Autodesk Inventor part; units mm, degrees
ref_plane "作業平面1" through (-36, -24, 0) normal (0, 0, 1) x (1, 0, 0)
ref_plane "作業平面2" through (-39.3, -27.3, -10) normal (0, 0, 1) x (1, 0, 0)
ref_plane "作業平面3" through (-36, -24, -2) normal (0, 0, -1) x (0, 1, 0)
sketch "スケッチ1" plane through (0, 0, 0) normal (0, 0, 1) x (1, 0, 0)
  line L0 (36, 24) -> (36, -24) construction
  line L1 (-36, 24) -> (36, 24) construction
  line L2 (-36, -24) -> (-36, 24) construction
  line L3 (36, -24) -> (-36, -24) construction
  circle A0 centre (-33, 21) radius 1.5 construction
  circle A1 centre (-33, -21) radius 1.5 construction
  circle A2 centre (33, 21) radius 1.5 construction
  circle A3 centre (33, -21) radius 1.5 construction
  line L4 (-36.3, 24.3) -> (36.3, 24.3)
  line L5 (36.3, 24.3) -> (36.3, -24.3)
  line L6 (36.3, -24.3) -> (-36.3, -24.3)
  line L7 (-36.3, -24.3) -> (-36.3, 24.3)
  circle A4 centre (-33, -21) radius 1.6
  circle A5 centre (-33, 21) radius 1.6
  circle A6 centre (33, -21) radius 1.6
  circle A7 centre (33, 21) radius 1.6
  line L8 (-39.3, 27.3) -> (39.3, 27.3)
  line L9 (39.3, 27.3) -> (39.3, -27.3)
  line L10 (39.3, -27.3) -> (-39.3, -27.3)
  line L11 (-39.3, -27.3) -> (-39.3, 27.3)
  line L12 (-36.3, -14.3) -> (-26.3, -14.3)
  line L13 (-26.3, -14.3) -> (-26.3, -24.3)
  line L14 (-55.02, 0) -> (55.02, 0) construction
  line L15 (0, -38.22) -> (0, 38.22) construction
  line L16 (-36.3, 14.3) -> (-26.3, 14.3)
  line L17 (-26.3, 14.3) -> (-26.3, 24.3)
  line L18 (36.3, -14.3) -> (26.3, -14.3)
  line L19 (26.3, -14.3) -> (26.3, -24.3)
  line L20 (26.3, 14.3) -> (26.3, 24.3)
  line L21 (36.3, 14.3) -> (26.3, 14.3)
  line L22 (22, 5) -> (29, 5) construction
  line L23 (29, -5) -> (22, -5) construction
  line L24 (36, 24) -> (36, -24)
  line L25 (36, -24) -> (-36, -24)
  line L26 (-36, -24) -> (-36, 24)
  line L27 (-36, 24) -> (36, 24)
  circle A8 centre (-33, 21) radius 1.5
  circle A9 centre (-33, -21) radius 1.5
  circle A10 centre (33, 21) radius 1.5
  circle A11 centre (33, -21) radius 1.5
  line L28 (39.3, 5) -> (36.3, 5)
  line L29 (39.3, -5) -> (36.3, -5)
  circle A12 centre (33, 21) radius 3
  circle A13 centre (33, -21) radius 3
  circle A14 centre (-33, 21) radius 3
  circle A15 centre (-33, -21) radius 3
  point P0 (0, 0)
  dimension "d0" = 0.3
  dimension "d1" = 3.2
  dimension "d2" = 3
  dimension "d7" = 10
  dimension "d16" = 6
extrude "押し出し1" add sketch "スケッチ1" along normal blind 7 and the other way blind 3 contours L7 L6 L5 L29 L9 L10 L11 L8 L28 L4 | L28 L9 L29 L5
ref_plane "作業平面1" through (-36, -24, 0) normal (0, 0, 1) x (1, 0, 0)
extrude "押し出し3" add sketch "スケッチ1" against normal up to surface (7 mm away) from surface at 7 contours L4 L17 L27 L26 L16 L7 | L4 L5 L21 L24 L27 L20 | L17 L16 L26 A14 L27 | L12 L26 L25 L13 L6 L7 | L27 A12 L24 L21 L20 | A14 L26 L27 | A14 | L12 L13 L25 A15 L26 | L27 L24 A12 | A12 | A15 L25 L26 | A15 | L19 L25 L24 L18 L5 L6 | L24 A13 L25 L19 L18 | A13 | L24 L25 A13
extrude "押し出し4" add sketch "スケッチ1" along normal blind 3 from surface at 7 contours L7 L6 L5 L29 L9 L10 L11 L8 L28 L4 | L4 L17 L27 L26 L16 L7 | L4 L20 L27 L17 | L16 L26 L12 L7 | L4 L5 L21 L24 L27 L20 | L27 L20 L21 L24 L18 L19 L25 L13 L12 L26 L16 L17 | L17 L16 L26 A14 L27 | L12 L26 L25 L13 L6 L7 | L27 A12 L24 L21 L20 | A14 L26 L27 | A14 | L12 L13 L25 A15 L26 | L5 L18 L24 L21 | L27 L24 A12 | A12 | L13 L25 L19 L6 | A15 L25 L26 | A15 | L28 L9 L29 L5 | L19 L25 L24 L18 L5 L6 | L24 A13 L25 L19 L18 | A13 | L24 L25 A13
ref_plane "作業平面2" through (-39.3, -27.3, -10) normal (0, 0, 1) x (1, 0, 0)
ref_plane "作業平面3" through (-36, -24, -2) normal (0, 0, -1) x (0, 1, 0)
sketch "スケッチ4" plane through (0, 0, 0) normal (0, 0, 1) x (1, 0, 0)
  line L0 (36.3, 24.3) -> (36.3, -24.3)
  line L1 (39.3, 27.3) -> (39.3, -27.3)
  line L2 (39.3, 5) -> (36.3, 5)
  line L3 (39.3, -5) -> (36.3, -5)
  point P0 (0, 0)
extrude "押し出し5" cut sketch "スケッチ4" along normal up to surface (8 mm away) from surface at -10
sketch "スケッチ5" plane through (-39.3, -27.3, 10) normal (0, 0, 1) x (1, 0, 0)
  circle A0 centre (6.3, 6.3) radius 3
  circle A1 centre (72.3, 6.3) radius 3
  circle A2 centre (72.3, 48.3) radius 3
  circle A3 centre (6.3, 48.3) radius 3
  line L0 (0, 0) -> (0, 54.6)
  line L1 (78.6, 0) -> (0, 0)
  line L2 (78.6, 54.6) -> (78.6, 0)
  line L3 (0, 54.6) -> (78.6, 54.6)
  circle A4 centre (72.3, 6.3) radius 1.6
  circle A5 centre (6.3, 6.3) radius 1.6
  circle A6 centre (6.3, 48.3) radius 1.6
  circle A7 centre (72.3, 48.3) radius 1.6
  point P0 (39.3, 27.3)
extrude "押し出し6" add sketch "スケッチ5" along normal blind 5 contours L0 L3 L2 L1
fillet "フィレット1" radius 5 4 edges at (-39.3, 27.3, 6) (-39.3, -27.3, 6) (39.3, 27.3, 6) (39.3, -27.3, 6)
properties part number "enclosure"
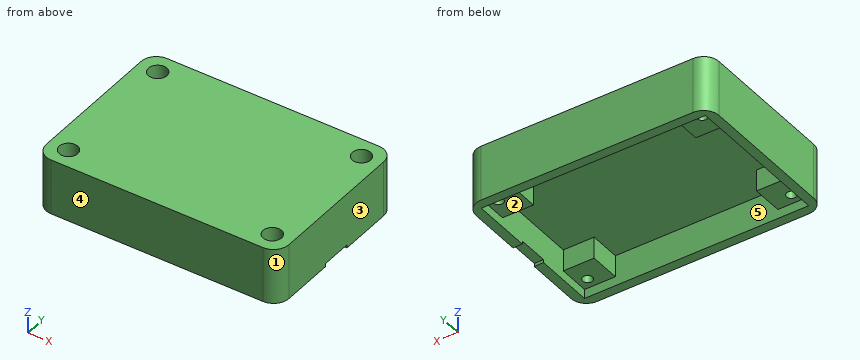
Part model, mm, in its own coordinate system. Face numbers are marked on the shaded views. A direction names the side the tool comes from. Coordinates: 2 decimals unless noted, no trailing zeros. Order: outer loops, then holes, each group sorted by start corner. A loop starts at its lowest first (then second) coordinate and runs counter-clockwise, first axis right, second up. Notation, with made-up numbers: M 88.25,1.25 L 118.25,1.25 A23 ccw 118.25,32.25 Z; hole C -10.5,43.25 d10. An arc over 180 degrees is marked long. Use a Markdown table: item, result.
(1) Cut at D-D on z = 13.75. Write the cut outline in (x, y), then the cut area to 3 significant figures.
A:
| item | result |
|---|---|
| outline | M -39.3,-22.3 A5 ccw -34.3,-27.3 L 34.3,-27.3 A5 ccw 39.3,-22.3 L 39.3,22.3 A5 ccw 34.3,27.3 L -34.3,27.3 A5 ccw -39.3,22.3 Z; hole C -33,-21 d6; hole C -33,21 d6; hole C 33,-21 d6; hole C 33,21 d6 |
| area | 4,160 mm^2 |
(2) Cut at C-C on x = 33. Write the cut outline in (y, z), then the cut area to 3 significant figures.
A:
| item | result |
|---|---|
| outline | M -27.3,-3 L -24.3,-3 L -24.3,0 L -22.6,0 L -22.6,10 L -24,10 L -24,15 L -27.3,15 Z; M -19.4,0 L -14.3,0 L -14.3,7 L 14.3,7 L 14.3,0 L 19.4,0 L 19.4,10 L 18,10 L 18,15 L -18,15 L -18,10 L -19.4,10 Z; M 22.6,0 L 24.3,0 L 24.3,-3 L 27.3,-3 L 27.3,15 L 24,15 L 24,10 L 22.6,10 Z |
| area | 513 mm^2 |
(3) Cut at B-B on z = 2.75. Write the cut outline in (x, y).
A:
| item | result |
|---|---|
| outline | M -39.3,-22.3 A5 ccw -34.3,-27.3 L 34.3,-27.3 A5 ccw 39.3,-22.3 L 39.3,22.3 A5 ccw 34.3,27.3 L -34.3,27.3 A5 ccw -39.3,22.3 Z; hole M -36.3,-14.3 L -26.3,-14.3 L -26.3,-24.3 L 26.3,-24.3 L 26.3,-14.3 L 36.3,-14.3 L 36.3,14.3 L 26.3,14.3 L 26.3,24.3 L -26.3,24.3 L -26.3,14.3 L -36.3,14.3 Z; hole C -33,-21 d3.2; hole C -33,21 d3.2; hole C 33,-21 d3.2; hole C 33,21 d3.2 |
(4) Probe L1, parallel to Y at x = -33, z = 6.25; L2, parallel to Y at x = 33, z = 13.1; L3, parallel to Y at x = -7.5, z = 5. List the from-to ranges inside material, lowest first.
A:
| item | result |
|---|---|
| L1 | y = -27.3 to -22.6, -19.4 to -14.3, 14.3 to 19.4, 22.6 to 27.3 |
| L2 | y = -27.3 to -24, -18 to 18, 24 to 27.3 |
| L3 | y = -27.3 to -24.3, 24.3 to 27.3 |
(5) Tool access for the marked faces 1 and 2: list every direction of +Z, -Z, +X, -X, +Y, -Y with a clear straight run to the whole face (end or side of a thin tool).
A:
| item | result |
|---|---|
| face 1 | +Z, -Z, +X, -Y |
| face 2 | -Z |
(6) Pull direction X, two halves, no side cores. Call the marked faces 3, 4 and 5: released by +X, released by -X, zero draft, split by the parting line, or undercut.
A:
| item | result |
|---|---|
| face 3 | released by +X |
| face 4 | zero draft |
| face 5 | undercut |
(7) Cut at A-A on y = 21. Write the cut outline in (x, z).
A:
| item | result |
|---|---|
| outline | M -39.3,-3 L -36.3,-3 L -36.3,0 L -34.6,0 L -34.6,10 L -36,10 L -36,15 L -39.3,15 Z; M -31.4,0 L -26.3,0 L -26.3,7 L 26.3,7 L 26.3,0 L 31.4,0 L 31.4,10 L 30,10 L 30,15 L -30,15 L -30,10 L -31.4,10 Z; M 34.6,0 L 36.3,0 L 36.3,-3 L 39.3,-3 L 39.3,15 L 36,15 L 36,10 L 34.6,10 Z |
(8) Flat gauge pins, fed straight in: pin 1 (10 mm diameter, centred on x = 12, y = 7.5, fed in from -Z); pin 2 (0.8 mm diameter, centred on x = 37, z = -2.5, fed in from +Y); pin 3 (5 mm diameter, centred on x = -33, y = -21, fed in from -Z). Where does each tip first touch, or does it go through?
A:
| item | result |
|---|---|
| pin 1 | stops at z = 7 |
| pin 2 | stops at y = 26.74 |
| pin 3 | stops at z = 0 |
